Here's how the part is built. I have some questions about the finished solid (model axes, mm). Face numbers are marked on the shaded views. A direction names the side the tool comes from. Round coordinates to 2 decimals unless told otherwise and drop trailing zeros. Order: outer loops, then holes, each group sorted by start corner. A loop starts at its lowest first (then second) coordinate and runs counter-clockwise, first axis right, second up. Notation, with made-up numbers: (66, 82.5) - (82, 82.5) arc R15 cw to (82, 95.5) - close; hole circle Ø10 at (-19.5, 27.25). An arc over 180 degrees is marked (long way). One line per item, written item: value.
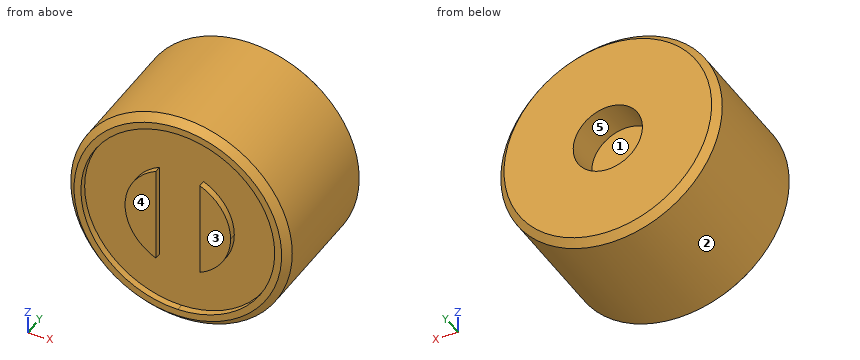
from build123d import *

# Parameters (mm, degrees)
SKETCH1_R           = 3.2
BOSS_EXTRUDE1_DEPTH = 4
CHAMFER1_SIZE       = 0.2
SKETCH2_R           = 1
CUT_EXTRUDE1_DEPTH  = 1
CUT_EXTRUDE2_DEPTH  = 0.2


with BuildPart() as part:
    # Sketch1 → Boss-Extrude1 (new body)
    with BuildSketch(Plane(origin=(0, 0, 0), x_dir=(1, 0, 0), z_dir=(0, 1, 0))):
        with Locations(Location((0, 0, 0), (0, 0, 270))):
            Circle(SKETCH1_R)
    extrude(amount=BOSS_EXTRUDE1_DEPTH)

    # Chamfer1
    chamfer1_edges = [part.edges().sort_by_distance(p)[0] for p in [
        (0, 0, -3.2),
        (0, 4, -3.2),
    ]]
    chamfer(chamfer1_edges, length=CHAMFER1_SIZE)

    # Sketch2 → Cut-Extrude1 (cut)
    with BuildSketch(Plane(origin=(0, 4, 0), x_dir=(1, 0, 0), z_dir=(0, 1, 0))):
        with Locations(Location((0, 0, 0), (0, 0, 270))):
            Circle(SKETCH2_R)
    extrude(amount=-CUT_EXTRUDE1_DEPTH, mode=Mode.SUBTRACT)

    # Sketch3 → Cut-Extrude2 (cut)
    with BuildSketch(Plane.XZ):
        with BuildLine():
            ThreePointArc((2.8, 0), (1.979898987, 1.979898987), (0, 2.8))
            Line((0, 2.8), (0, 1.525))
            ThreePointArc((0, 1.525), (0.324963643, 1.489974373), (0.635, 1.386506401))
            ThreePointArc((0.635, 1.386506401), (1.283354978, 0.823786987), (1.525, 0))
            ThreePointArc((1.525, 0), (1.283354978, -0.823786987), (0.635, -1.386506401))
            ThreePointArc((0.635, -1.386506401), (0.324963643, -1.489974373), (0, -1.525))
            Line((0, -1.525), (0, -2.8))
            ThreePointArc((0, -2.8), (1.979898987, -1.979898987), (2.8, 0))
        make_face()
        with BuildLine():
            Line((0, 1.525), (0, 2.8))
            ThreePointArc((0, 2.8), (-2.8, 0), (0, -2.8))
            Line((0, -2.8), (0, -1.525))
            ThreePointArc((0, -1.525), (-0.324963643, -1.489974373), (-0.635, -1.386506401))
            ThreePointArc((-0.635, -1.386506401), (-1.525, 0), (-0.635, 1.386506401))
            ThreePointArc((-0.635, 1.386506401), (-0.324963643, 1.489974373), (0, 1.525))
        make_face()
        with BuildLine():
            Line((0, -1.525), (0, 1.525))
            ThreePointArc((0, 1.525), (-0.324963643, 1.489974373), (-0.635, 1.386506401))
            Line((-0.635, 1.386506401), (-0.635, -1.386506401))
            ThreePointArc((-0.635, -1.386506401), (-0.324963643, -1.489974373), (0, -1.525))
        make_face()
        with BuildLine():
            ThreePointArc((0.635, 1.386506401), (0.324963643, 1.489974373), (0, 1.525))
            Line((0, 1.525), (0, -1.525))
            ThreePointArc((0, -1.525), (0.324963643, -1.489974373), (0.635, -1.386506401))
            Line((0.635, -1.386506401), (0.635, 1.386506401))
        make_face()
    extrude(amount=-CUT_EXTRUDE2_DEPTH, mode=Mode.SUBTRACT)


solid = part.part
Q1. If I drill on line 1 along X through (y, z) = (3.25, 0); line 2 along X through (y, z) = (3.85, 0); line 3 along Y through (x, z) = (0.5, 1.5), over which ranges is the centre line in solid material (lowest first)?
Results list:
line 1: -3.2 to -1, 1 to 3.2
line 2: -3.15 to -1, 1 to 3.15
line 3: 0.2 to 4
Q2. We'd pull the mould along Z, two halves only. Please class the marked faces 1, 2 and 3: released by +Z, released by -Z, zero draft, split by the parting line, or undercut.
Results list:
face 1: undercut
face 2: split by the parting line
face 3: zero draft
Q3. Will this pin go through, and if not, where does the flat tip stop? pin 1 (1.5 mm diameter, centred on y = 2, z = -1.5, fed in from -X).
Results list:
pin 1: x = -3.11
Q4. If we section it at B-B, the plane y = 0.3: Please give me the cut outline in (x, z).
Results list:
outline: circle Ø6.4 at (0, 0)
Q5. If we section it at A-A, the plane y = 3.55: Please give me the cut outline in (x, z), then the cut area to 3 significant figures.
Results list:
outline: circle Ø6.4 at (0, 0); hole circle Ø2 at (0, 0)
area: 29.0 mm²
Q6. Which directions (+Z, -Z, +X, -X, +Y, -Y) give clear straight access to the entire face, cutting with the end or side of a thin tool? Please do the marked faces 4 and 5.
Results list:
face 4: +Z, -Z, +X, -X, -Y
face 5: +Y
